Verification items for the finished model (mm, model axes). A direction names the side the tool comes from. Give positions to 0.01 mm unless a question says otherwise; leave off trailing zeros. Order: outer loops, then holes, each group sorted by start corner. A loop starts at its lowest first (then second) coordinate and runs counter-clockwise, first axis right, second up.
from build123d import *

# Parameters (mm, degrees)
SKETCH_W        = 18.7
SKETCH_H        = 35.7
PAD_DEPTH       = 17
SKETCH001_W     = 14.5
SKETCH001_H     = 31.5
POCKET_DEPTH    = 7
SKETCH002_W     = 14.5
SKETCH002_H     = 8
SKETCH002_H_2   = 4
POCKET001_DEPTH = 10.001
SKETCH003_R     = 0.75
SKETCH003_W     = 7
SKETCH003_H     = 7
POCKET002_DEPTH = 5
SKETCH004_W     = 18.7
SKETCH004_H     = 11.1
SKETCH004_W_2   = 14.5
SKETCH004_H_2   = 4
PAD001_DEPTH    = 25
CHAMFER_SIZE    = 1


with BuildPart() as part:
    # Sketch → Pad (new body)
    with BuildSketch(Plane.XZ):
        with Locations((0, 11.75)):
            Rectangle(SKETCH_W, SKETCH_H)
    extrude(amount=PAD_DEPTH)

    # Sketch001 (on Face6 of Pad) → Pocket (cut)
    with BuildSketch(Plane.XZ.offset(17)):
        with Locations((0, 11.75)):
            Rectangle(SKETCH001_W, SKETCH001_H)
    extrude(amount=-POCKET_DEPTH, mode=Mode.SUBTRACT)

    # Sketch002 (on Face11 of Pocket) → Pocket001 (cut, through all)
    with BuildSketch(Plane.XZ.offset(10)):
        Rectangle(SKETCH002_W, SKETCH002_H)
        with Locations((0, 25.5)):
            Rectangle(SKETCH002_W, SKETCH002_H_2)
    extrude(amount=-POCKET001_DEPTH, mode=Mode.SUBTRACT)

    # Sketch003 (on Face9 of Pocket001) → Pocket002 (cut)
    with BuildSketch(Plane.XZ.offset(10)):
        with Locations((0, 20.5)):
            Circle(SKETCH003_R)
        with Locations((-3.75, 11.5)):
            Rectangle(SKETCH003_W, SKETCH003_H)
    extrude(amount=-POCKET002_DEPTH, mode=Mode.SUBTRACT)

    # Sketch004 (on Face4 of Pocket002) → Pad001 (join)
    with BuildSketch(Plane(origin=(0, 0, 0), x_dir=(1, 0, 0), z_dir=(0, 1, 0))):
        with Locations((0, -24.05)):
            Rectangle(SKETCH004_W, SKETCH004_H)
        with Locations((0, -25.5)):
            Rectangle(SKETCH004_W_2, SKETCH004_H_2, mode=Mode.SUBTRACT)
    extrude(amount=PAD001_DEPTH)

    # Chamfer
    chamfer_edges = [part.edges().sort_by_distance(p)[0] for p in [
        (0, -17, 29.6),
        (9.35, -17, 11.75),
        (9.35, 4, 29.6),
        (-9.35, 4, 29.6),
        (-9.35, -17, 11.75),
        (0, -17, -6.1),
        (9.35, -8.5, -6.1),
        (-9.35, -8.5, -6.1),
        (0, 0, -6.1),
        (9.35, 0, 6.2),
        (9.35, 12.5, 18.5),
        (9.35, 25, 24.05),
        (-9.35, 25, 24.05),
        (-9.35, 12.5, 18.5),
        (-9.35, 0, 6.2),
        (0, 25, 18.5),
        (0, 25, 29.6),
        (0, -10, 23.5),
        (0, -10, 4),
        (-0.75, -10, 20.5),
        (-3.75, -10, 15),
        (-0.25, -10, 11.5),
        (-3.75, -10, 8),
    ]]
    chamfer(chamfer_edges, length=CHAMFER_SIZE)


solid = part.part
(1) Go/stop test with flat-tipped pins: pin 1 (8.5 mm diameter, centred on x = -2.5, z = 8.5, fed in from +Y); pin 2 (1.4 mm diameter, centred on x = 0, z = 20.5, fed in from -Y); pin 3 (5.5 mm diameter, centred on x = -3.5, z = 10, fed in from -Y). Record where each tip stops, or that it passes through.
Solved:
pin 1: stops at y = 0
pin 2: stops at y = -5
pin 3: stops at y = -9.75
(2) Release check for a two-part mould opening along Z. For faces 1 (the flat face through (-8.84, -0.49, 7.03)), 2 (the flat face through (-8.65, -0.62, -5.42)), 3 (the flat face through (-0.1, -9.5, 23)) record: pulls with the +Z half, pulls with the -Z half, needs draft (parallel to the pull), parting line crosses it, or undercut.
Solved:
face 1: needs draft
face 2: pulls with the -Z half
face 3: undercut
(3) Section check C-C, the plane z = 26. Enter the section's corners in (x, y).
Solved:
outline: (-9.35, -16) - (-8.35, -17) - (-7.25, -17) - (-7.25, 25) - (-8.35, 25) - (-9.35, 24) - close; (7.25, -17) - (8.35, -17) - (9.35, -16) - (9.35, 24) - (8.35, 25) - (7.25, 25) - close
(4) Set-up check for faces 4 (the flat face through (0, 0, 9)), 5 (the flat face through (0, -8, -6.1)), 6 (the flat face through (-8.73, -16.3, 28.92)), 7 (the flat face through (0, 8, 23.5)), 8 (the cylindrical face through (-0.163, -7.028, 19.768)): record each of +Z, -Z, +X, -X, +Y, -Y from which the full face is reachable in a straight line by a thin tool's end or side.
Solved:
face 4: -Z, +X, -X, +Y
face 5: -Z, +X, -X, +Y, -Y
face 6: +Z, -X, -Y
face 7: +Y, -Y
face 8: -Y
(5) Section check A-A, the plane y = -7.5. Enter the section's corners in (x, z), then the cut area to 3 significant figures.
Solved:
outline: (-9.35, -5.1) - (-8.35, -6.1) - (8.35, -6.1) - (9.35, -5.1) - (9.35, 28.6) - (8.35, 29.6) - (-8.35, 29.6) - (-9.35, 28.6) - close; hole (-7.25, -4) - (7.25, -4) - (7.25, 4) - (-7.25, 4) - close; hole (-7.25, 8) - (-0.25, 8) - (-0.25, 15) - (-7.25, 15) - close; hole (-7.25, 23.5) - (7.25, 23.5) - (7.25, 27.5) - (-7.25, 27.5) - close; hole circle Ø1.5 at (0, 20.5)
area: 441 mm2
(6) Section check B-B, the plane x = -4. Enter the section's corners in (y, z), then the cut area to 3 significant figures.
Solved:
outline: (-17, -5.1) - (-16, -6.1) - (-1, -6.1) - (0, -5.1) - (0, -4) - (-17, -4) - close; (-17, 27.5) - (25, 27.5) - (25, 28.6) - (24, 29.6) - (-16, 29.6) - (-17, 28.6) - close; (-10, 5) - (-9, 4) - (0, 4) - (0, 18.5) - (24, 18.5) - (25, 19.5) - (25, 23.5) - (-9, 23.5) - (-10, 22.5) - (-10, 16) - (-9, 15) - (-5, 15) - (-5, 8) - (-9, 8) - (-10, 7) - close
area: 404 mm2
(7) Scan lines: line 1 (Z direction, x = 0, y = -6.85); line 2 (Z direction, x = 2, y = 2); line 3 (Y direction, x = -6.5, z = 7). Record each from-to range of solid material in increasing order.
Solved:
line 1: z = -6.1 to -4, 4 to 19.75, 21.25 to 23.5, 27.5 to 29.6
line 2: z = 18.5 to 23.5, 27.5 to 29.6
line 3: y = -10 to 0
(8) Section check D-D, the plane y = 2. Enter the section's corners in (x, z), then the cut area to 3 significant figures.
Solved:
outline: (-9.35, 19.5) - (-8.35, 18.5) - (8.35, 18.5) - (9.35, 19.5) - (9.35, 28.6) - (8.35, 29.6) - (-8.35, 29.6) - (-9.35, 28.6) - close; hole (-7.25, 23.5) - (7.25, 23.5) - (7.25, 27.5) - (-7.25, 27.5) - close
area: 148 mm2
